```python
from build123d import *

# Parameters (mm, degrees)
SKETCH1_R           = 17
BOSS_EXTRUDE1_DEPTH = 25
SKETCH2_R           = 19
BOSS_EXTRUDE2_DEPTH = 8
BOSS_EXTRUDE3_DEPTH = 12
SKETCH6_R           = 16
BOSS_EXTRUDE4_DEPTH = 15


with BuildPart() as part:
    # Sketch1 → Boss-Extrude1 (new body)
    with BuildSketch(Plane.XY):
        Circle(SKETCH1_R)
    extrude(amount=BOSS_EXTRUDE1_DEPTH)

    # Sketch2 → Boss-Extrude2 (add)
    with BuildSketch(Plane.XY):
        Circle(SKETCH2_R)
    extrude(amount=-BOSS_EXTRUDE2_DEPTH)

    # Sketch5 → Boss-Extrude3 (add)
    with BuildSketch(Plane(origin=(0, 0, -8), x_dir=(-1, 0, 0), z_dir=(0, 0, -1))):
        with BuildLine():
            ThreePointArc((44, -13.416407865), (0, -46), (-44, -13.416407865))
            ThreePointArc((-44, -13.416407865), (-33.683444249, 16.469257624), (-13.668094758, 40.943123461))
            ThreePointArc((-13.668094758, 40.943123461), (0, 46), (13.668094758, 40.943123461))
            ThreePointArc((13.668094758, 40.943123461), (33.683444249, 16.469257624), (44, -13.416407865))
        make_face()
    extrude(amount=BOSS_EXTRUDE3_DEPTH)

    # Sketch6 → Boss-Extrude4 (add)
    with BuildSketch(Plane(origin=(0, 0, -20), x_dir=(-1, 0, 0), z_dir=(0, 0, -1))):
        with Locations((0, 25)):
            Circle(SKETCH6_R)
    extrude(amount=BOSS_EXTRUDE4_DEPTH)

    # Mirror2: part across plane


with BuildPart() as part_1:
    add(part.part)
    add(part.part.mirror(Plane(origin=(0, 25, -35), x_dir=(1, 0, 0), z_dir=(0, 0, -1))))


solid = part_1.part
```
Here's how the part is built. I have some questions about the finished solid (model axes, mm). A direction names the side the tool comes from. Coordinates: 2 decimals unless noted, no trailing zeros. Order: outer loops, then holes, each group sorted by start corner. A loop starts at its lowest first (then second) coordinate and runs counter-clockwise, first axis right, second up.
Item 1: If we section it at D-D, the plane z = -52.5: List the corners of the cut face in (x, y) for me.
Response values:
outline: (-44, -13.42) arc R46 ccw to (44, -13.42) arc R90 ccw to (13.67, 40.94) arc R21 ccw to (-13.67, 40.94) arc R90 ccw to start
Item 2: Thinking about a two-plate mould opening in Z: for faces 1 (the face through (-1, -20, -62)), 2 (the face through (-1, -10, -20)), 3 (the face through (0, 46, -56)), 4 (the face through (-1, -10, -50)), which applies, pulls with the +Z half, pulls with the -Z half, needs draft (parallel to the pull), parting line crosses it, or undercut?
Response values:
face 1: pulls with the -Z half
face 2: undercut
face 3: needs draft
face 4: undercut
Item 3: If we section it at C-C, the plane x = 0: List the corners of the cut face in (y, z) for me, then the cut area to 3 significant figures.
Response values:
outline: (-46, -62) - (-19, -62) - (-19, -70) - (-17, -70) - (-17, -95) - (17, -95) - (17, -70) - (19, -70) - (19, -62) - (46, -62) - (46, -50) - (41, -50) - (41, -20) - (46, -20) - (46, -8) - (19, -8) - (19, 0) - (17, 0) - (17, 25) - (-17, 25) - (-17, 0) - (-19, 0) - (-19, -8) - (-46, -8) - (-46, -20) - (9, -20) - (9, -50) - (-46, -50) - close
area: 5,480 mm2
Item 4: I need wall thicknesses on probe 1 along Z at (x, y) = (26, -4.5); probe 2 along Z at (x, y) = (7.5, 9); probe 3 along Z at (x, y) = (9, 26.5). Which ranges of each line are inside material? Lowest first, please.
Response values:
probe 1: z = -62 to -50, -20 to -8
probe 2: z = -95 to -50, -20 to 25
probe 3: z = -62 to -8
Item 5: If we section it at B-B, the plane y = 0: List the corners of the cut face in (x, z) for me, then the cut area to 3 significant figures.
Response values:
outline: (-40.82, -62) - (-19, -62) - (-19, -70) - (-17, -70) - (-17, -95) - (17, -95) - (17, -70) - (19, -70) - (19, -62) - (40.82, -62) - (40.82, -50) - (-40.82, -50) - close; (-40.82, -20) - (40.82, -20) - (40.82, -8) - (19, -8) - (19, 0) - (17, 0) - (17, 25) - (-17, 25) - (-17, 0) - (-19, 0) - (-19, -8) - (-40.82, -8) - close
area: 4,270 mm2
Item 6: Which directions (+Z, -Z, +X, -X, +Y, -Y) give clear straight access to the entire face, cutting with the end or side of a thin tool? Please do faces 5 (the face through (-0.821, -45.993, -56.084)), 6 (the face through (8.767, -16.856, -3.944)), 7 (the face through (9.139, 14.334, -82.325)).
Response values:
face 5: +Z, -Z, -Y
face 6: +Z
face 7: -Z
Item 7: I'm going to push flat-ended pins straight in: pin 1 Ø10 at (x, z) = (-23, 8.5) entering from +Y; pin 2 Ø5 at (x, y) = (20, 15.5) entering from +Z; pin 3 Ø1 at (x, z) = (-35, -50.5) entering from +Y; pin 4 Ø1 at (x, z) = (-34.5, -11.5) entering from +Y. Where does each tip first touch, or does it pass through?
Response values:
pin 1: passes through
pin 2: stops at z = -8
pin 3: stops at y = 14.97
pin 4: stops at y = 15.9
Item 8: If we section it at A-A, the plane x = 37.5: List the corners of the cut face in (y, z) for me.
Response values:
outline: (-26.64, -62) - (8.79, -62) - (8.79, -50) - (-26.64, -50) - close; (-26.64, -20) - (8.79, -20) - (8.79, -8) - (-26.64, -8) - close
